from build123d import *

# Parameters (mm, degrees)
EXTRUDE001_DEPTH       = 9
BOX001_W               = 200
BOX001_H               = 200
BOX001_DEPTH           = 200
BOX001_PLACEMENT_ANGLE = 45
BOX_W                  = 200
BOX_H                  = 200
BOX_DEPTH              = 200
BOX_PLACEMENT_ANGLE    = 45
EXTRUDE_DEPTH          = 440
FILLET001_R            = 1
FILLET_R               = 1
FUSION_PLACEMENT_ANGLE = 90


with BuildPart() as extrude001:
    # Sketch001 → Extrude001 (new body)
    with BuildSketch(Plane.XY):
        Polygon((-75, 0), (-69.803848, 9), (100, 9), (100, 0), align=None)
    extrude(amount=EXTRUDE001_DEPTH)


with BuildPart() as extrude001_1:
    # Extrude001 placement: moved
    add(extrude001.part.moved(Location((0, 0, 215.5))))


with BuildPart() as cube001:
    # Box001 → Box001 (new body)
    with BuildSketch(Plane.XY):
        with Locations((100, 100)):
            Rectangle(BOX001_W, BOX001_H)
    extrude(amount=BOX001_DEPTH)


with BuildPart() as cube001_1:
    # Box001 placement: moved
    add(cube001.part.moved(Location((-96, 139.726, 300.357))).rotate(Axis((-96, 139.726, 300.357), (1, 0, 0)), BOX001_PLACEMENT_ANGLE))


with BuildPart() as cube:
    # Box → Box (new body)
    with BuildSketch(Plane.XY):
        with Locations((100, 100)):
            Rectangle(BOX_W, BOX_H)
    extrude(amount=BOX_DEPTH)


with BuildPart() as cube_1:
    # Box placement: moved
    add(cube.part.moved(Location((-96, 141.421356, -141.421356))).rotate(Axis((-96, 141.421356, -141.421356), (1, 0, 0)), BOX_PLACEMENT_ANGLE))


with BuildPart() as cut001:
    # Sketch → Extrude (new body)
    with BuildSketch(Plane.XY):
        Polygon((-75, 0), (0, 129.903811), (75, 0), align=None)
    extrude(amount=EXTRUDE_DEPTH)

    # Cut: cut Cube
    add(cube_1.part, mode=Mode.SUBTRACT)

    # Cut001: cut Cube001
    add(cube001_1.part, mode=Mode.SUBTRACT)


with BuildPart() as fillet001:
    # Fillet001 base: copy of Cut001
    add(cut001.part)

    # Fillet001
    fillet001_edges = [fillet001.edges().sort_by_distance(p)[0] for p in [
        (-37.5, 64.951905, 64.951905),
        (0, 129.903811, 220.0415),
        (-37.47604, 64.993405, 375.089595),
        (37.5, 64.951905, 64.951905),
        (37.47604, 64.993405, 375.089595),
    ]]
    fillet(fillet001_edges, radius=FILLET001_R)


with BuildPart() as fillet001_1:
    # Fillet001 placement: moved
    add(fillet001.part.moved(Location((0, -3, 0))))


with BuildPart() as fusion:
    # Fillet base: copy of Cut001
    add(cut001.part)

    # Fillet
    fillet_edges = [fusion.edges().sort_by_distance(p)[0] for p in [
        (-37.5, 64.951905, 64.951905),
        (0, 129.903811, 220.0415),
        (-37.47604, 64.993405, 375.089595),
        (37.5, 64.951905, 64.951905),
        (37.47604, 64.993405, 375.089595),
    ]]
    fillet(fillet_edges, radius=FILLET_R)

    # Cut002: cut Fillet001
    add(fillet001_1.part, mode=Mode.SUBTRACT)

    # Fusion: union Extrude001
    add(extrude001_1.part)


with BuildPart() as fusion_1:
    # Fusion placement: moved
    add(fusion.part.moved(Location((-105.5, -15.92, 333))).rotate(Axis((-105.5, -15.92, 333), (0, 1, 0)), FUSION_PLACEMENT_ANGLE))


solid = fusion_1.part
Check sheet for the modelled part. Datum: model origin and axes. Units: mm. A direction names the side the tool comes from. Round coordinates to 2 decimals unless told otherwise and drop trailing zeros. Loops run counter-clockwise (first coordinate to the right, second up) from the corner with the lowest first, then second, coordinate; pieces in that order, holes last. Notation, with made-up numbers: (68, 3) -> (78, 3) arc R5 cw to (78, 10) -> close; hole circle Ø8 at (71.5, 35). An arc over 180 degrees is marked (long way). Put each result on its own line as item: value. Start each with the question number.
1. Scan lines: probe 1 along Z at (x, y) = (215, 70); probe 2 along Z at (x, y) = (85.5, 42.5); probe 3 along X at (y, z) = (18.5, 386). Record each from-to range of solid material in increasing order.
2. Access from +Z, -Z, +X, -X, +Y, -Y to the whole of each face (thin tool, end or side, straight path). Record for faces 1 (the face through (114, -6.92, 248)), 2 (the face through (269.12, 49.29, 370.15)), 3 (the face through (-52.77, 33.81, 334.02)).
3. Gauge pin test, flat ends, axial feed: pin 1 (10 mm diameter, centred on x = 114, z = 340.5, fed in from +Y); pin 2 (1 mm diameter, centred on x = 50.5, z = 294, fed in from +Y); pin 3 (6 mm diameter, centred on x = 166.5, z = 299, fed in from +Y). Record the tip position at first contact, or that the pin passes through.
4. Section check A-A (x = 174.5). Enter the section's corners in (y, z), plus the area to 3 significant figures.
5. Draft check along Z on faces 4 (the face through (-40.339, 45.997, 295.69)), 5 (the face through (283.617, 35.046, 334.039)), 6 (the face through (-40.05, 49.272, 370.162)). Enter one of: +Z half, -Z half, draft (parallel to the pull), parting line (faces both ways), or undercut.
Findings:
1. probe 1: z = 307.61 to 309.34, 356.66 to 358.39
1. probe 2: z = 291.73 to 293.46, 372.54 to 374.27
1. probe 3: x = -71.08 to -67.99, 297.07 to 300.16
2. face 1: -Z, +X, -X, +Y
2. face 2: +Z, +X, +Y
2. face 3: -Y
3. pin 1: stops at y = 109.65
3. pin 2: stops at y = 47.3
3. pin 3: stops at y = 60.29
4. outline: (-15.92, 258) -> (112.48, 332.13) arc R1 ccw to (112.48, 333.87) -> (-15.92, 408) -> (-15.92, 406.27) -> (109.48, 333.87) arc R1 cw to (109.48, 332.13) -> (-15.92, 259.73) -> close
4. area: 445 mm^2
5. face 4: undercut
5. face 5: draft
5. face 6: +Z half
